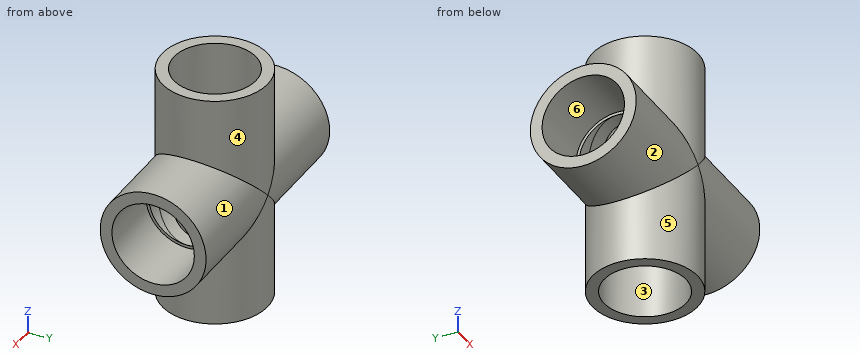
from build123d import *
from build123d import SkipClean  # not in build123d's __all__

# Parameters (mm, degrees)
F0_R     = 14.2875
F0_R_2   = 11.1125
F1_DEPTH = 31.75
F0_R_3   = 10.31875
F2_DEPTH = 14.2875
F3_R     = 14.2875
F3_R_2   = 11.1125
F4_DEPTH = 31.75
F3_R_3   = 10.31875
F5_DEPTH = 14.2875
F6_DEPTH = 14.2875
F7_DEPTH = 14.2875


with BuildPart() as f1:
    # F0 (on Top) → F1 (new body, symmetric)
    with BuildSketch(Plane.XY):
        Circle(F0_R)
        Circle(F0_R_2, mode=Mode.SUBTRACT)
    extrude(amount=F1_DEPTH, both=True)

    # F0 (on Top) → F2 (join, symmetric)
    with BuildSketch(Plane.XY):
        Circle(F0_R_2)
        Circle(F0_R_3, mode=Mode.SUBTRACT)
    extrude(amount=F2_DEPTH, both=True)

    # F3 (on Right) → F4 (join, symmetric)
    with BuildSketch(Plane.YZ):
        Circle(F3_R)
        Circle(F3_R_2, mode=Mode.SUBTRACT)
    extrude(amount=F4_DEPTH, both=True)

    # F3 (on Right) → F5 (join, symmetric)
    with BuildSketch(Plane.YZ):
        Circle(F3_R_2)
        Circle(F3_R_3, mode=Mode.SUBTRACT)
    with SkipClean():  # cleaning this boolean's faces spoils the solid; the shape is the same uncleaned
        extrude(amount=F5_DEPTH, both=True)

    # F0 (on Top) → F6 (cut, symmetric)
    with BuildSketch(Plane.XY):
        Circle(F0_R_3)
    with SkipClean():  # cleaning this boolean's faces spoils the solid; the shape is the same uncleaned
        extrude(amount=F6_DEPTH, both=True, mode=Mode.SUBTRACT)

    # F3 (on Right) → F7 (cut, symmetric)
    with BuildSketch(Plane.YZ):
        Circle(F3_R_3)
    extrude(amount=F7_DEPTH, both=True, mode=Mode.SUBTRACT)


solid = f1.part
CAD build for the part. Positions are in the model's coordinates, mm. Face numbers are marked on the shaded views. A direction names the side the tool comes from. Give positions to 0.01 mm unless a question says otherwise; leave off trailing zeros. Loops run counter-clockwise (first coordinate to the right, second up) from the corner with the lowest first, then second, coordinate; pieces in that order, holes last. Notation, with made-up numbers: M 78.25,39.5 L 113.25,39.5 A31 cw 113.25,78.5 Z; hole C -33.75,63.25 d6. An arc over 180 degrees is marked long. Answer in a Markdown table with one row per item. Add a question column.
Item 1: Tool access for the marked faces 1, 2, 3 and 4: list every direction of +Z, -Z, +X, -X, +Y, -Y with a clear straight run to the whole face (end or side of a thin tool).
Item 2: Mould opens along Y. For the marked faces 5 and 6 say: +Y half, -Y half, draft (parallel to the pull), parting line (faces both ways), or undercut.
Item 3: Band-saw the part on C-C on x = -17. Give the cut face in (y, z) (1 decimal).
Item 4: Drop flat-ended pins along their axis: P1, Ø10, axis at x = 9.5, z = -11.5, coming from the -Y side; P2, Ø11, axis at y = -5, z = -1, coming from the +X side; P3, Ø13.5, axis at y = 0, z = 0, coming from the -X side; P4, Ø12, axis at x = 21, z = -17.5, coming from the +Y side. Give the stop position or say it passes through.
Item 5: Probe probe 1 along Y at (x, z) = (0, -28); probe 2 along Y at (x, z) = (0, 6). List the from-to ranges inside material, lowest first.
Reply:
| question | item | result |
|---|---|---|
| 1 | face 1 | +X |
| 1 | face 2 | -X |
| 1 | face 3 | -Z |
| 1 | face 4 | +Z |
| 2 | face 5 | parting line |
| 2 | face 6 | undercut |
| 3 | outline | C 0,0 d28.6; hole C 0,0 d22.2 |
| 4 | P1 | stops at y = -13.56 |
| 4 | P2 | stops at x = 14.29 |
| 4 | P3 | passes through |
| 4 | P4 | stops at y = 8.48 |
| 5 | probe 1 | y = -14.29 to -11.11, 11.11 to 14.29 |
| 5 | probe 2 | y = -14.29 to -10.32, 10.32 to 14.29 |
